Verification items for the finished model (mm, model axes). A direction names the side the tool comes from. Give positions to 0.01 mm unless a question says otherwise; leave off trailing zeros. Loops run counter-clockwise (first coordinate to the right, second up) from the corner with the lowest first, then second, coordinate; pieces in that order, holes last. Notation, with made-up numbers: M -36.75,-39.5 L -28.75,-39.5 A25 ccw -28.75,-24.5 Z; hole C 84,4 d8. An arc over 180 degrees is marked long. Answer in a Markdown table with one row per item.
```python
from build123d import *

# Parameters (mm, degrees)
SKETCH1_W           = 136
SKETCH1_H           = 46
SKETCH1_R           = 1.05
BOSS_EXTRUDE1_DEPTH = 3
CUT_EXTRUDE1_REACH  = 5
SKETCH4_W           = 3
SKETCH4_H           = 9
SKETCH4_H_2         = 7
SKETCH4_W_2         = 10
SKETCH4_H_3         = 3
SKETCH4_W_3         = 11


with BuildPart() as part:
    # Sketch1 → Boss-Extrude1 (new body)
    with BuildSketch(Plane.XY):
        with Locations((68, 23)):
            Rectangle(SKETCH1_W, SKETCH1_H)
        with Locations((88, 20.5)):
            Circle(SKETCH1_R, mode=Mode.SUBTRACT)
        with Locations((48, 20.5)):
            Circle(SKETCH1_R, mode=Mode.SUBTRACT)
        with Locations((48, 3.5)):
            Circle(SKETCH1_R, mode=Mode.SUBTRACT)
        with Locations((88, 3.5)):
            Circle(SKETCH1_R, mode=Mode.SUBTRACT)
    extrude(amount=BOSS_EXTRUDE1_DEPTH)

    # Sketch4 → Cut-Extrude1 (cut, up to next)
    with BuildSketch(Plane.XY.offset(3), mode=Mode.PRIVATE) as cut_extrude1_sk1:
        Polygon((0, 46), (0, 43), (3, 43), (10, 43), (10, 46), align=None)
    cut_extrude1_tool1 = extrude(cut_extrude1_sk1.sketch, amount=-CUT_EXTRUDE1_REACH, mode=Mode.PRIVATE) & part.part
    add(cut_extrude1_tool1.solids().sort_by_distance((5, 44.5, 3))[0], mode=Mode.SUBTRACT)
    # Sketch4 → Cut-Extrude1 (cut, up to next)
    with BuildSketch(Plane.XY.offset(3), mode=Mode.PRIVATE) as cut_extrude1_sk2:
        with Locations((1.5, 38.5)):
            Rectangle(SKETCH4_W, SKETCH4_H)
    cut_extrude1_tool2 = extrude(cut_extrude1_sk2.sketch, amount=-CUT_EXTRUDE1_REACH, mode=Mode.PRIVATE) & part.part
    add(cut_extrude1_tool2.solids().sort_by_distance((1.5, 38.5, 3))[0], mode=Mode.SUBTRACT)
    # Sketch4 → Cut-Extrude1 (cut, up to next)
    with BuildSketch(Plane.XY.offset(3), mode=Mode.PRIVATE) as cut_extrude1_sk3:
        with Locations((1.5, 20.5)):
            Rectangle(SKETCH4_W, SKETCH4_H)
    cut_extrude1_tool3 = extrude(cut_extrude1_sk3.sketch, amount=-CUT_EXTRUDE1_REACH, mode=Mode.PRIVATE) & part.part
    add(cut_extrude1_tool3.solids().sort_by_distance((1.5, 20.5, 3))[0], mode=Mode.SUBTRACT)
    # Sketch4 → Cut-Extrude1 (cut, up to next)
    with BuildSketch(Plane.XY.offset(3), mode=Mode.PRIVATE) as cut_extrude1_sk4:
        with Locations((1.5, 3.5)):
            Rectangle(SKETCH4_W, SKETCH4_H_2)
    cut_extrude1_tool4 = extrude(cut_extrude1_sk4.sketch, amount=-CUT_EXTRUDE1_REACH, mode=Mode.PRIVATE) & part.part
    add(cut_extrude1_tool4.solids().sort_by_distance((1.5, 3.5, 3))[0], mode=Mode.SUBTRACT)
    # Sketch4 → Cut-Extrude1 (cut, up to next)
    with BuildSketch(Plane.XY.offset(3), mode=Mode.PRIVATE) as cut_extrude1_sk5:
        with Locations((25, 44.5)):
            Rectangle(SKETCH4_W_2, SKETCH4_H_3)
    cut_extrude1_tool5 = extrude(cut_extrude1_sk5.sketch, amount=-CUT_EXTRUDE1_REACH, mode=Mode.PRIVATE) & part.part
    add(cut_extrude1_tool5.solids().sort_by_distance((25, 44.5, 3))[0], mode=Mode.SUBTRACT)
    # Sketch4 → Cut-Extrude1 (cut, up to next)
    with BuildSketch(Plane.XY.offset(3), mode=Mode.PRIVATE) as cut_extrude1_sk6:
        with Locations((45, 44.5)):
            Rectangle(SKETCH4_W_2, SKETCH4_H_3)
    cut_extrude1_tool6 = extrude(cut_extrude1_sk6.sketch, amount=-CUT_EXTRUDE1_REACH, mode=Mode.PRIVATE) & part.part
    add(cut_extrude1_tool6.solids().sort_by_distance((45, 44.5, 3))[0], mode=Mode.SUBTRACT)
    # Sketch4 → Cut-Extrude1 (cut, up to next)
    with BuildSketch(Plane.XY.offset(3), mode=Mode.PRIVATE) as cut_extrude1_sk7:
        with Locations((65.5, 44.5)):
            Rectangle(SKETCH4_W_3, SKETCH4_H_3)
    cut_extrude1_tool7 = extrude(cut_extrude1_sk7.sketch, amount=-CUT_EXTRUDE1_REACH, mode=Mode.PRIVATE) & part.part
    add(cut_extrude1_tool7.solids().sort_by_distance((65.5, 44.5, 3))[0], mode=Mode.SUBTRACT)
    # Sketch4 → Cut-Extrude1 (cut, up to next)
    with BuildSketch(Plane.XY.offset(3), mode=Mode.PRIVATE) as cut_extrude1_sk8:
        with Locations((91, 44.5)):
            Rectangle(SKETCH4_W_2, SKETCH4_H_3)
    cut_extrude1_tool8 = extrude(cut_extrude1_sk8.sketch, amount=-CUT_EXTRUDE1_REACH, mode=Mode.PRIVATE) & part.part
    add(cut_extrude1_tool8.solids().sort_by_distance((91, 44.5, 3))[0], mode=Mode.SUBTRACT)
    # Sketch4 → Cut-Extrude1 (cut, up to next)
    with BuildSketch(Plane.XY.offset(3), mode=Mode.PRIVATE) as cut_extrude1_sk9:
        with Locations((111, 44.5)):
            Rectangle(SKETCH4_W_2, SKETCH4_H_3)
    cut_extrude1_tool9 = extrude(cut_extrude1_sk9.sketch, amount=-CUT_EXTRUDE1_REACH, mode=Mode.PRIVATE) & part.part
    add(cut_extrude1_tool9.solids().sort_by_distance((111, 44.5, 3))[0], mode=Mode.SUBTRACT)
    # Sketch4 → Cut-Extrude1 (cut, up to next)
    with BuildSketch(Plane.XY.offset(3), mode=Mode.PRIVATE) as cut_extrude1_sk10:
        Polygon((133, 43), (136, 43), (136, 46), (126, 46), (126, 43), align=None)
    cut_extrude1_tool10 = extrude(cut_extrude1_sk10.sketch, amount=-CUT_EXTRUDE1_REACH, mode=Mode.PRIVATE) & part.part
    add(cut_extrude1_tool10.solids().sort_by_distance((131, 44.5, 3))[0], mode=Mode.SUBTRACT)
    # Sketch4 → Cut-Extrude1 (cut, up to next)
    with BuildSketch(Plane.XY.offset(3), mode=Mode.PRIVATE) as cut_extrude1_sk11:
        with Locations((134.5, 38.5)):
            Rectangle(SKETCH4_W, SKETCH4_H)
    cut_extrude1_tool11 = extrude(cut_extrude1_sk11.sketch, amount=-CUT_EXTRUDE1_REACH, mode=Mode.PRIVATE) & part.part
    add(cut_extrude1_tool11.solids().sort_by_distance((134.5, 38.5, 3))[0], mode=Mode.SUBTRACT)
    # Sketch4 → Cut-Extrude1 (cut, up to next)
    with BuildSketch(Plane.XY.offset(3), mode=Mode.PRIVATE) as cut_extrude1_sk12:
        with Locations((134.5, 20.5)):
            Rectangle(SKETCH4_W, SKETCH4_H)
    cut_extrude1_tool12 = extrude(cut_extrude1_sk12.sketch, amount=-CUT_EXTRUDE1_REACH, mode=Mode.PRIVATE) & part.part
    add(cut_extrude1_tool12.solids().sort_by_distance((134.5, 20.5, 3))[0], mode=Mode.SUBTRACT)
    # Sketch4 → Cut-Extrude1 (cut, up to next)
    with BuildSketch(Plane.XY.offset(3), mode=Mode.PRIVATE) as cut_extrude1_sk13:
        with Locations((134.5, 3.5)):
            Rectangle(SKETCH4_W, SKETCH4_H_2)
    cut_extrude1_tool13 = extrude(cut_extrude1_sk13.sketch, amount=-CUT_EXTRUDE1_REACH, mode=Mode.PRIVATE) & part.part
    add(cut_extrude1_tool13.solids().sort_by_distance((134.5, 3.5, 3))[0], mode=Mode.SUBTRACT)


solid = part.part
```
Item 1: Scan lines: L1, parallel to Y at x = 88, z = 1.5; L2, parallel to X at y = 24, z = 2.05; L3, parallel to Y at x = 91.5, z = 1.15. Record each from-to range of solid material in increasing order. Write a range as [from, to].
Reported:
| item | result |
|---|---|
| L1 | y = [0, 2.45], [4.55, 19.45], [21.55, 43] |
| L2 | x = [3, 133] |
| L3 | y = [0, 43] |
Item 2: Release check for a two-part mould opening along Y. For faces 1 (the flat face through (67, 23, 0)), 2 (the flat face through (65, 43, 2)), 3 (the flat face through (1, 25, 2)) record: released by +Y, released by -Y, zero draft, split by the parting line, or undercut.
Reported:
| item | result |
|---|---|
| face 1 | zero draft |
| face 2 | released by +Y |
| face 3 | undercut |
Item 3: Sectioned sample at C-C (y = 36). Record the cut outline in (x, z), and give its area (3 significant figures).
Reported:
| item | result |
|---|---|
| outline | M 3,0 L 133,0 L 133,3 L 3,3 Z |
| area | 390 mm^2 |
Item 4: Sectioned sample at A-A (z = 0.85). State how many separate pieces and enclosed holes the cut face has, and give its area (3 significant figures).
Reported:
| item | result |
|---|---|
| separate pieces | 1 |
| enclosed holes | 4 |
| area | 5,880 mm^2 |
Item 5: Sectioned sample at B-B (x = 108). Record the cut outline in (y, z), and give its area (3 significant figures).
Reported:
| item | result |
|---|---|
| outline | M 0,0 L 43,0 L 43,3 L 0,3 Z |
| area | 129 mm^2 |
Item 6: Go/stop test with flat-tipped pins: pin 1 (1.7 mm diameter, centred on x = 48, y = 20.5, fed in from -Z); pin 2 (0.9 mm diameter, centred on y = 44, z = 1.5, fed in from +X); pin 3 (1 mm diameter, centred on y = 20.5, z = 0.5, fed in from -X); pin 4 (1.5 mm diameter, centred on y = 44.5, z = 2, fed in from -X). Record where each tip stops, or that it passes through.
Reported:
| item | result |
|---|---|
| pin 1 | passes through |
| pin 2 | stops at x = 126 |
| pin 3 | stops at x = 3 |
| pin 4 | stops at x = 10 |
Item 7: Tool access check on faces 4 (the flat face through (3, 20, 2)), 5 (the flat face through (134, 34, 2)), 6 (the flat face through (1, 7, 2)). Record the directions out of +Z, -Z, +X, -X, +Y, -Y that give a thin tool (end or side, any length) a straight path to the whole face; none if there is none.
Reported:
| item | result |
|---|---|
| face 4 | +Z, -Z, -X |
| face 5 | +Z, -Z, +X, +Y |
| face 6 | +Z, -Z, -X, -Y |
